Model file for the job. Use its own axes, mm. A direction names the side the tool comes from. Coordinates: 2 decimals unless noted, no trailing zeros. Write each loop counter-clockwise with the first axis right and the second up, starting at its lowest first coordinate (ties: lowest second). Pieces come first, ordered by that corner, then holes. Notation, with made-up numbers: M 66.25,63.25 L 95.25,63.25 A28 cw 95.25,101.25 Z; hole C 72.5,88 d8. An arc over 180 degrees is marked long. One line per question, with ' | ' between items. Start each with the question number.
(1) Cut at C-C (z = 25). Write the cut outline in (x, y).
(2) Wall check: probe 1 along Y at (x, z) = (3, 41); probe 2 along X at (y, z) = (-6, 46); probe 3 along Z at (x, y) = (-16, -16). Give the ranges that are in metal, low to high.
(3) Cut at B-B (y = -36). Write the cut outline in (x, z), plus the area to 3 significant figures.
(4) Two-plate mould, pull along Y, no slides. Class faces 3 (the face through (78.74, -1, 26)), 4 (the face through (-1, 50.8, 32)), 5 (the face through (-1, -53.34, 26)), 6 (the face through (76.2, -1, 32)): +Y half, -Y half, draft (parallel to the pull), parting line (faces both ways), or undercut.
(5) Flat gauge pins, fed straight in: pin 1 Ø3 at (x, y) = (52.5, -17.5) entering from +Z; pin 2 Ø1.3 at (x, y) = (77, 11) entering from -Z. Where does each tip first touch, or does it go through?
(6) Tool access for faces 1 (the face through (0, 52, 53.34)), 2 (the face through (-1, 1, 9.144)): list every direction of +Z, -Z, +X, -X, +Y, -Y with a clear straight run to the whole face (end or side of a thin tool).
(7) Cut at D-D (y = 23). Write the cut outline in (x, z).
(8) Cut at A-A (z = 45). Write the cut outline in (x, y).
from build123d import *

# Parameters (mm, degrees)
SKETCH1_W           = 157.48
SKETCH1_H           = 106.68
BOSS_EXTRUDE1_DEPTH = 53.34
SKETCH3_W           = 152.4
SKETCH3_H           = 101.6
CUT_EXTRUDE1_DEPTH  = 44.196
SKETCH4_W           = 8.89
SKETCH4_H           = 12.7
CUT_EXTRUDE2_DEPTH  = 43.18
SKETCH6_W           = 10.922
SKETCH6_H           = 14.224
CUT_EXTRUDE3_DEPTH  = 43.18
SKETCH7_W           = 9.525
SKETCH7_H           = 12.7
CUT_EXTRUDE4_DEPTH  = 12.7


with BuildPart() as part:
    # Sketch1 → Boss-Extrude1 (new body)
    with BuildSketch(Plane.XY):
        Rectangle(SKETCH1_W, SKETCH1_H)
    extrude(amount=BOSS_EXTRUDE1_DEPTH)

    # Sketch3 → Cut-Extrude1 (cut)
    with BuildSketch(Plane.XY.offset(53.34)):
        Rectangle(SKETCH3_W, SKETCH3_H)
    extrude(amount=-CUT_EXTRUDE1_DEPTH, mode=Mode.SUBTRACT)

    # Sketch4 → Cut-Extrude2 (cut)
    with BuildSketch(Plane(origin=(78.74, 0, 0), x_dir=(0, 0, -1), z_dir=(1, 0, 0))):
        with Locations((-32.385, -8.89)):
            Rectangle(SKETCH4_W, SKETCH4_H)
    extrude(amount=-CUT_EXTRUDE2_DEPTH, mode=Mode.SUBTRACT)

    # Sketch6 → Cut-Extrude3 (cut)
    with BuildSketch(Plane.ZY.offset(78.74)):
        with Locations((42.799, -39.878)):
            Rectangle(SKETCH6_W, SKETCH6_H)
    extrude(amount=-CUT_EXTRUDE3_DEPTH, mode=Mode.SUBTRACT)

    # Sketch7 → Cut-Extrude4 (cut)
    with BuildSketch(Plane(origin=(78.74, 0, 0), x_dir=(0, 0, -1), z_dir=(1, 0, 0))):
        with Locations((-43.4975, 13.97)):
            Rectangle(SKETCH7_W, SKETCH7_H)
    extrude(amount=-CUT_EXTRUDE4_DEPTH, mode=Mode.SUBTRACT)


solid = part.part
Filled in:
1) outline: M -78.74,-53.34 L 78.74,-53.34 L 78.74,53.34 L -78.74,53.34 Z; hole M -76.2,-50.8 L 76.2,-50.8 L 76.2,50.8 L -76.2,50.8 Z
2) probe 1: -53.34 to -50.8, 50.8 to 53.34 | probe 2: -78.74 to -76.2, 76.2 to 78.74 | probe 3: 0 to 9.14
3) outline: M -78.74,0 L 78.74,0 L 78.74,53.34 L 76.2,53.34 L 76.2,9.14 L -76.2,9.14 L -76.2,37.34 L -78.74,37.34 Z; M -78.74,48.26 L -76.2,48.26 L -76.2,53.34 L -78.74,53.34 Z | area: 1,640 mm²
4) face 3: draft | face 4: undercut | face 5: -Y half | face 6: undercut
5) pin 1: z = 9.14 | pin 2: z = 0
6) face 1: +Z, +X, -X, +Y, -Y | face 2: +Z
7) outline: M -78.74,0 L 78.74,0 L 78.74,53.34 L 76.2,53.34 L 76.2,9.14 L -76.2,9.14 L -76.2,53.34 L -78.74,53.34 Z
8) outline: M -78.74,-53.34 L 78.74,-53.34 L 78.74,7.62 L 76.2,7.62 L 76.2,-50.8 L -76.2,-50.8 L -76.2,-46.99 L -78.74,-46.99 Z; M -78.74,-32.77 L -76.2,-32.77 L -76.2,50.8 L 76.2,50.8 L 76.2,20.32 L 78.74,20.32 L 78.74,53.34 L -78.74,53.34 Z
